Autodesk Inventor part; units mm, degrees
ref_plane "YZ Plane" through (0, 0, 0) normal (1, 0, 0) x (0, 1, 0)
ref_plane "XZ Plane" through (0, 0, 0) normal (0, 1, 0) x (-1, 0, 0)
ref_plane "XY Plane" through (0, 0, 0) normal (0, 0, 1) x (1, 0, 0)
sketch "Sketch1" plane through (0, 0, 0) normal (0, 1, 0) x (-1, 0, 0)
  arc A0 (-6, 0) -> (6, 0) centre (0, 0) ccw
  arc A1 (-8, 0) -> (8, 0) centre (0, 0) ccw
  line L0 (-17, 0) -> (-17, -11.2563)
  line L1 (-17, -11.2563) -> (8, -11.2563)
  line L2 (8, -11.2563) -> (8, 0)
  line L3 (8, 0) -> (6, 0)
  line L4 (-6, 0) -> (-17, 0)
  line L5 (6, 0) -> (-6, 0) construction
  dimension "d0" = 12
  dimension "d1" = 16
  dimension "d2" = 8
  dimension "d3" = 9
extrude "Tykkelse" add sketch "Sketch1" along normal mid plane 12 contours A1 L2 L1 L0 L4
extrude "Lille cirkel" add sketch "Sketch1" along normal mid plane 6 contours A0 L3 A1 L4
sketch "Sketch2" plane through (17, 6, -11.2563) normal (0, 0, -1) x (-1, 0, 0)
  circle A0 centre (6, -6) radius 2
  line L0 (0, 0) -> (0, -12)
  line L1 (25, -12) -> (0, -12)
  point P0 (17, -6)
  dimension "d9" = 4
  dimension "d10" = 6
  dimension "d11" = 6
extrude "Monteringshul" cut sketch "Sketch2" against normal up to surface (11.2563 mm away)
properties part number "Holder"
Geometry check sheet. Reference: the model listing, model coordinates, mm. A direction names the side the tool comes from. Round coordinates to 2 decimals unless told otherwise and drop trailing zeros. Order: outer loops, then holes, each group sorted by start corner. A loop starts at its lowest first (then second) coordinate and runs counter-clockwise, first axis right, second up. Notation, with made-up numbers: (31, -7) - (87, -7) arc R28 ccw to (87, 20) - close; hole circle Ø11 at (28.5, 33.25). An arc over 180 degrees is marked (long way). Use a Markdown table: item, result. Add a question column.
1) Section check B-B (x = 11). Record the cut outline in (y, z).
2) Thickness scan on line 1 along Y through (x, z) = (11, -8.25); line 2 along X through (y, z) = (-0.5, -2.25); line 3 along X through (y, z) = (1.5, -4). Record the ranges inside material, lowest first.
3) Gauge pin test, flat ends, axial feed: P1, Ø4, axis at x = -3.5, z = -3, coming from the -Y side; P2, Ø2.5, axis at x = 0, z = -6, coming from the +Y side. Record the tip position at first contact, or that the pin passes through.
4) Section check C-C (z = -4.5). Record the cut outline in (x, y), then the cut area to 3 significant figures.
5) Section check A-A (y = 0). Record the cut outline in (x, z), then the cut area to 3 significant figures.
6) Section check D-D (x = 0). Record the cut outline in (y, z).
7) Set-up check for faces 1 (the flat face through (13, -1, 0)), 2 (the cylindrical face through (0, -5, -8)): record each of +Z, -Z, +X, -X, +Y, -Y from which the full face is reachable in a straight line by a thin tool's end or side.
8) Mould release check, pull along Y, two halves, no side actions. Record for faces 3 (the cylindrical face through (12.6, -1.2, -5.7)), 4 (the flat face through (1.2, 3, -6.1)), 5 (the flat face through (7, -6, -7)), 6 (the cylindrical face through (0, 4, -8)): released by +Y, released by -Y, zero draft, split by the parting line, or undercut.
Established:
| question | item | result |
|---|---|---|
| 1 | outline | (-6, -11.26) - (-2, -11.26) - (-2, 0) - (-6, 0) - close; (2, -11.26) - (6, -11.26) - (6, 0) - (2, 0) - close |
| 2 | line 1 | -6 to -2, 2 to 6 |
| 2 | line 2 | -8 to -5.56, 5.56 to 9.06, 12.94 to 17 |
| 2 | line 3 | -8 to -4.47, 4.47 to 9.68, 12.32 to 17 |
| 3 | P1 | y = -3 |
| 3 | P2 | y = 3 |
| 4 | outline | (-8, -6) - (-6.61, -6) - (-6.61, -3) - (-3.97, -3) - (-3.97, 3) - (-6.61, 3) - (-6.61, 6) - (-8, 6) - close; (3.97, -3) - (6.61, -3) - (6.61, -6) - (17, -6) - (17, 6) - (6.61, 6) - (6.61, 3) - (3.97, 3) - close; hole circle Ø4 at (11, 0) |
| 4 | area | 160 mm2 |
| 5 | outline | (-8, -11.26) - (9, -11.26) - (9, 0) - (6, 0) arc R6 cw to (-6, 0) - (-8, 0) - close; (13, -11.26) - (17, -11.26) - (17, 0) - (13, 0) - close |
| 5 | area | 180 mm2 |
| 6 | outline | (-6, -11.26) - (6, -11.26) - (6, -8) - (3, -8) - (3, -6) - (-3, -6) - (-3, -8) - (-6, -8) - close |
| 7 | face 1 | +Z, +X, -X, +Y, -Y |
| 7 | face 2 | +Z, -Y |
| 8 | face 3 | undercut |
| 8 | face 4 | released by +Y |
| 8 | face 5 | released by -Y |
| 8 | face 6 | zero draft |
